Print and shaded views of the part. All mm, measured from the part's lowest x, y and z. A direction names the side the tool comes from. Round coordinates to 2 decimals unless told otherwise and drop trailing zeros. Order: outer loops, then holes, each group sorted by start corner. A loop starts at its lowest first (then second) coordinate and runs counter-clockwise, first axis right, second up. Notation, with made-up numbers: M 4.5,-31 L 8.5,-31 A13 cw 8.5,-25 Z; hole C 32.5,-25 d4. An arc over 180 degrees is marked long. Write each question's results on one line, items separated by ' | '. Start each with the question number.
1. Band-saw the part on D-D, the plane y = 22.5. List the corners of the cut face in (x, z), then the cut area to 3 significant figures.
2. Band-saw the part on A-A, the plane x = 111.5. List the corners of the cut face in (y, z).
3. Drop flat-ended pins along their axis: pin 1 Ø2 at (y, z) = (18, 17) entering from -X; pin 2 Ø5 at (y, z) = (11, 63) entering from +X; pin 3 Ø7.5 at (x, y) = (117, 9.5) entering from -Z. Give the stop position or say it passes through.
4. Which spindle directions (+Z, -Z, +X, -X, +Y, -Y) get a long thin tool onto all of the face, cutting with end or side? Do the marked faces 4, 5 and 6. Say none if no direction does.
5. Probe L1, parallel to X at y = 5.5, z = 36; L2, parallel to Z at x = 16.5, y = 7; L3, parallel to X at y = 11.5, z = 10. List the from-to ranges inside material, lowest first. Write a range as [from, to].
6. Band-saw the part on B-B, the plane z = 39. List the corners of the cut face in (x, y), then the cut area to 3 significant figures.
7. Two-plate mould, pull along Z, no slides. Class the marked faces 1, 2 and 3: +Z half, -Z half, draft (parallel to the pull), parting line (faces both ways), or undercut.
8. Band-saw the part on C-C, the plane z = 11. List the corners of the cut face in (x, y), then the cut area to 3 significant figures.
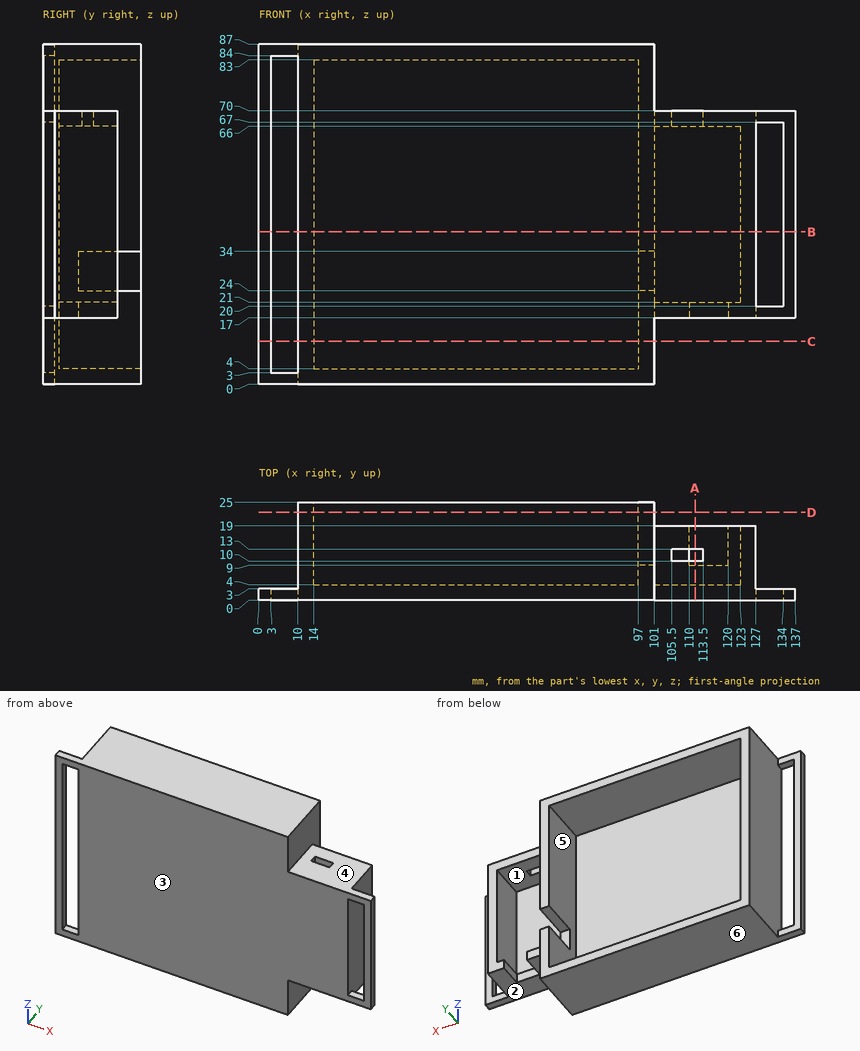
Solution:
1) outline: M 10,0 L 101,0 L 101,24 L 97,24 L 97,4 L 14,4 L 14,83 L 97,83 L 97,34 L 101,34 L 101,87 L 10,87 Z | area: 1,320 mm^2
2) outline: M 0,17 L 9,17 L 9,21 L 4,21 L 4,66 L 10,66 L 10,70 L 0,70 Z; M 13,66 L 19,66 L 19,70 L 13,70 Z
3) pin 1: x = 10 | pin 2: x = 127 | pin 3: z = 17
4) face 4: +Z, +X, +Y, -Y | face 5: +Y | face 6: -Z, +X, -X, +Y, -Y
5) L1: [10, 14], [97, 101], [123, 127] | L2: [0, 4], [83, 87] | L3: [10, 14], [97, 101]
6) outline: M 0,0 L 3,0 L 3,3 L 0,3 Z; M 10,0 L 127,0 L 127,19 L 123,19 L 123,4 L 101,4 L 101,25 L 97,25 L 97,4 L 14,4 L 14,25 L 10,25 Z; M 134,0 L 137,0 L 137,3 L 134,3 Z | area: 714 mm^2
7) face 1: undercut | face 2: -Z half | face 3: draft
8) outline: M 0,0 L 3,0 L 3,3 L 0,3 Z; M 10,0 L 101,0 L 101,25 L 97,25 L 97,4 L 14,4 L 14,25 L 10,25 Z | area: 541 mm^2
